Verification items for the finished model (mm, model axes). Coordinates: 2 decimals unless noted, no trailing zeros. Order: outer loops, then holes, each group sorted by start corner. A loop starts at its lowest first (then second) coordinate and runs counter-clockwise, first axis right, second up.
Q1. Cross-section at B-B, the plane y = 0. Record the boundary of the cut face in (x, z), and give its area (3 significant figures).
Q2. Thickness scan on line 1 (Y direction, x = 38, z = 1.25); line 2 (X direction, y = -10, z = 1); line 3 (Y direction, x = -37, z = 1.4). Record the ranges inside material, lowest first.
Q3. Cross-section at C-C, the plane x = -37. Record the boundary of the cut face in (y, z).
Q4. Cross-section at A-A, the plane x = 46. Record the boundary of the cut face in (y, z), and give its area (3 significant figures).
Q5. Depth check by flat-ended pin: P1, Ø2.5, axis at x = -45, y = 11.5, coming from the +Z side. Enter the tip coordinate at first touch or a pass-through.
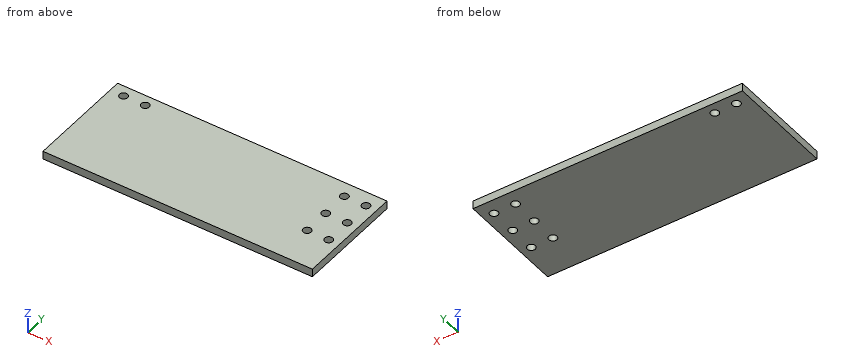
from build123d import *

# Parameters (mm, degrees)
SKETCH1_W           = 100
SKETCH1_H           = 55
SKETCH1_R           = 1.5
BOSS_EXTRUDE1_DEPTH = 3
SKETCH2_W           = 100
SKETCH2_H           = 12
CUT_EXTRUDE1_DEPTH  = 58.142366069
SKETCH3_W           = 100
SKETCH3_H           = 3
CUT_EXTRUDE2_DEPTH  = 58.142366069
SKETCH4_R           = 1.5
CUT_EXTRUDE3_DEPTH  = 56.760649207


with BuildPart() as part:
    # Sketch1 → Boss-Extrude1 (new body)
    with BuildSketch(Plane.XY):
        Rectangle(SKETCH1_W, SKETCH1_H)
        with Locations((38, 10)):
            Circle(SKETCH1_R, mode=Mode.SUBTRACT)
        with Locations((46, 10)):
            Circle(SKETCH1_R, mode=Mode.SUBTRACT)
        with Locations(Location((46, -10, 0), (0, 0, 180))):
            Circle(SKETCH1_R, mode=Mode.SUBTRACT)
        with Locations(Location((38, -10, 0), (0, 0, 180))):
            Circle(SKETCH1_R, mode=Mode.SUBTRACT)
        with Locations((38, 0)):
            Circle(SKETCH1_R, mode=Mode.SUBTRACT)
        with Locations((46, 0)):
            Circle(SKETCH1_R, mode=Mode.SUBTRACT)
    extrude(amount=BOSS_EXTRUDE1_DEPTH)

    # Sketch2 → Cut-Extrude1 (cut, through all)
    with BuildSketch(Plane.XY.offset(3)):
        with Locations((0, 21.5)):
            Rectangle(SKETCH2_W, SKETCH2_H)
    extrude(amount=-CUT_EXTRUDE1_DEPTH, mode=Mode.SUBTRACT)

    # Sketch3 → Cut-Extrude2 (cut, through all)
    with BuildSketch(Plane.XY.offset(3)):
        with Locations((0, -26)):
            Rectangle(SKETCH3_W, SKETCH3_H)
    extrude(amount=-CUT_EXTRUDE2_DEPTH, mode=Mode.SUBTRACT)

    # Sketch4 → Cut-Extrude3 (cut, through all)
    with BuildSketch(Plane.XY.offset(3)):
        with Locations((-45, 11.5)):
            Circle(SKETCH4_R)
        with Locations((-37, 11.5)):
            Circle(SKETCH4_R)
    extrude(amount=-CUT_EXTRUDE3_DEPTH, mode=Mode.SUBTRACT)


solid = part.part
Check values:
1. outline: (-50, 0) - (36.5, 0) - (36.5, 3) - (-50, 3) - close; (39.5, 0) - (44.5, 0) - (44.5, 3) - (39.5, 3) - close; (47.5, 0) - (50, 0) - (50, 3) - (47.5, 3) - close
1. area: 282 mm2
2. line 1: y = -24.5 to -11.5, -8.5 to -1.5, 1.5 to 8.5, 11.5 to 15.5
2. line 2: x = -50 to 36.5, 39.5 to 44.5, 47.5 to 50
2. line 3: y = -24.5 to 10, 13 to 15.5
3. outline: (-24.5, 0) - (10, 0) - (10, 3) - (-24.5, 3) - close; (13, 0) - (15.5, 0) - (15.5, 3) - (13, 3) - close
4. outline: (-24.5, 0) - (-11.5, 0) - (-11.5, 3) - (-24.5, 3) - close; (-8.5, 0) - (-1.5, 0) - (-1.5, 3) - (-8.5, 3) - close; (1.5, 0) - (8.5, 0) - (8.5, 3) - (1.5, 3) - close; (11.5, 0) - (15.5, 0) - (15.5, 3) - (11.5, 3) - close
4. area: 93.0 mm2
5. P1: passes through
